Can you work these out from the model? Positions are in its coordinate system, mm. Face numbers are marked on the shaded views. Round coordinates to 2 decimals unless told otherwise and drop trailing zeros. Loops run counter-clockwise (first coordinate to the right, second up) from the corner with the lowest first, then second, coordinate; pieces in that order, holes last. Notation, with made-up numbers: (-31, 2) -> (-4, 2) arc R16 cw to (-4, 26) -> close; hole circle Ø6 at (88.25, -16). An arc over 180 degrees is marked (long way). Answer as a JSON object with one key per item and string values.
```python
from build123d import *

# Parameters (mm, degrees)
PAD009_DEPTH          = 2
SKETCH015_R           = 2
POCKET005_DEPTH       = 2
POCKET006_DEPTH       = 2
PAD010_DEPTH          = 160
POLARPATTERN001_COUNT = 6
SKETCH018_W           = 8
SKETCH018_H           = 3
POCKET007_DEPTH       = 2
POLARPATTERN002_COUNT = 6
SKETCH019_W           = 14
SKETCH019_H           = 27
PAD011_DEPTH          = 3
POLARPATTERN003_COUNT = 6
POCKET008_DEPTH       = 5
POLARPATTERN004_COUNT = 6
SKETCH021_R           = 50
SKETCH021_R_2         = 46
PAD012_DEPTH          = 6
SKETCH022_W           = 4
SKETCH022_H           = 3
POCKET009_DEPTH       = 6
POLARPATTERN005_COUNT = 4
SKETCH023_W           = 2.5
SKETCH023_H           = 3
POLARPATTERN006_COUNT = 4
POCKET010_DEPTH       = 5


with BuildPart() as part:
    # Sketch014 → Pad009 (new body)
    with BuildSketch(Plane.XY):
        with BuildLine():
            Line((-52, -60), (52, -60))
            ThreePointArc((52, -60), (57.6568542495, -57.6568542495), (60, -52))
            Line((60, -52), (60, 52))
            ThreePointArc((60, 52), (57.6568542495, 57.6568542495), (52, 60))
            Line((52, 60), (-52, 60))
            ThreePointArc((-52, 60), (-57.6568542495, 57.6568542495), (-60, 52))
            Line((-60, 52), (-60, -52))
            ThreePointArc((-60, -52), (-57.6568542495, -57.6568542495), (-52, -60))
        make_face()
    extrude(amount=PAD009_DEPTH)

    # Sketch015 (on Face10 of Pad009) → Pocket005 (cut)
    with BuildSketch(Plane.XY.offset(2)):
        with Locations((-52, 52)):
            Circle(SKETCH015_R)
        with Locations((52, 52)):
            Circle(SKETCH015_R)
        with Locations((52, -52)):
            Circle(SKETCH015_R)
        with Locations((-52, -52)):
            Circle(SKETCH015_R)
    extrude(amount=-POCKET005_DEPTH, mode=Mode.SUBTRACT)

    # Sketch016 (on Face5 of Pocket005) → Pocket006 (cut)
    with BuildSketch(Plane.XY.offset(2)):
        Polygon((30, 0), (15, 25.9807621135), (-15, 25.9807621135), (-30, 0), (-15, -25.9807621135), (15, -25.9807621135), align=None)
    extrude(amount=-POCKET006_DEPTH, mode=Mode.SUBTRACT)

    # Sketch017 (on Face5 of Pocket006) → Pad010 (join)
    with BuildSketch(Plane.XY.offset(2)):
        Polygon((-7, 26), (7, 26), (7, 29), (5, 29), (5, 27.5), (-5, 27.5), (-5, 29), (-7, 29), align=None)
    pad010 = extrude(amount=PAD010_DEPTH)

    # PolarPattern001: Pad010 ×6 about axis
    polarpattern001_axis = Axis((0, 0, 2), (0, 0, 1))
    for i in range(1, POLARPATTERN001_COUNT):
        add(pad010.rotate(polarpattern001_axis, i * 360 / POLARPATTERN001_COUNT))

    # Sketch018 (on Face5 of PolarPattern001) → Pocket007 (cut)
    with BuildSketch(Plane.XY.offset(2)):
        with Locations((0, 30)):
            Rectangle(SKETCH018_W, SKETCH018_H)
    pocket007 = extrude(amount=-POCKET007_DEPTH, mode=Mode.SUBTRACT)

    # PolarPattern002: Pocket007 ×6 about axis
    polarpattern002_axis = Axis((0, 0, 2), (0, 0, 1))
    for i in range(1, POLARPATTERN002_COUNT):
        add(pocket007.rotate(polarpattern002_axis, i * 360 / POLARPATTERN002_COUNT), mode=Mode.SUBTRACT)

    # Sketch019 (on Face98 of PolarPattern002) → Pad011 (join)
    with BuildSketch(Plane.XY.offset(162)):
        with Locations((0, 13.5)):
            Rectangle(SKETCH019_W, SKETCH019_H)
    pad011 = extrude(amount=-PAD011_DEPTH)

    # PolarPattern003: Pad011 ×6 about axis
    polarpattern003_axis = Axis((0, 0, 162), (0, 0, 1))
    for i in range(1, POLARPATTERN003_COUNT):
        add(pad011.rotate(polarpattern003_axis, i * 360 / POLARPATTERN003_COUNT))

    # Sketch020 (on Face71 of PolarPattern003) → Pocket008 (cut)
    with BuildSketch(Plane(origin=(23.8156986041, 13.75, 0), x_dir=(-0.5, 0.8660254038, 0), z_dir=(0.8660254038, 0.5, 0))):
        Polygon((2.9997494237, 155.3827539752), (1.5334536671, 158), (-1.4662957566, 158.0387736377), (-2.9997494237, 155.4603012506), (-1.5334536671, 152.8430552259), (1.4662957566, 152.8042815882), align=None)
    pocket008 = extrude(amount=-POCKET008_DEPTH, mode=Mode.SUBTRACT)

    # PolarPattern004: Pocket008 ×6 about axis
    polarpattern004_axis = Axis((0, 0, 0), (0, 0, 1))
    for i in range(1, POLARPATTERN004_COUNT):
        add(pocket008.rotate(polarpattern004_axis, i * 360 / POLARPATTERN004_COUNT), mode=Mode.SUBTRACT)

    # Sketch021 (on Face5 of PolarPattern004) → Pad012 (join)
    with BuildSketch(Plane.XY.offset(2)):
        Circle(SKETCH021_R)
        Circle(SKETCH021_R_2, mode=Mode.SUBTRACT)
    extrude(amount=PAD012_DEPTH)

    # Sketch022 (on Face47 of Pad012) → Pocket009 (cut)
    with BuildSketch(Plane.XY.offset(8)):
        with Locations((0, -49)):
            Rectangle(SKETCH022_W, SKETCH022_H)
    pocket009 = extrude(amount=-POCKET009_DEPTH, mode=Mode.SUBTRACT)

    # PolarPattern005: Pocket009 ×4 about axis
    polarpattern005_axis = Axis((0, 0, 8), (0, 0, 1))
    for i in range(1, POLARPATTERN005_COUNT):
        add(pocket009.rotate(polarpattern005_axis, i * 360 / POLARPATTERN005_COUNT), mode=Mode.SUBTRACT)

    # SubtractivePipe: sweep along a path in Sketch024
    with BuildLine(Plane.XY.offset(2)) as subtractivepipe_path:
        ThreePointArc((-12.940932525, -48.2962966011), (-6.5262994853, -49.5722444018), (0, -50))
    # Sketch023 (on DatumPlane) → SubtractivePipe (sweep, cut)
    with BuildSketch(Plane.YZ.offset(-2)):
        with Locations((-48.7099839872, 3.5)):
            Rectangle(SKETCH023_W, SKETCH023_H)
    subtractivepipe = sweep(path=subtractivepipe_path.line, mode=Mode.SUBTRACT)

    # PolarPattern006: SubtractivePipe ×4 about axis
    polarpattern006_axis = Axis((0, 0, 0), (0, 0, 1))
    for i in range(1, POLARPATTERN006_COUNT):
        add(subtractivepipe.rotate(polarpattern006_axis, i * 360 / POLARPATTERN006_COUNT), mode=Mode.SUBTRACT)

    # Sketch025 (on Face123 of PolarPattern006) → Pocket010 (cut)
    with BuildSketch(Plane.XY.offset(162)):
        Polygon((6.9282031151, 4.0000001994), (-2.303e-07, 8), (-6.9282033454, 3.9999998006), (-6.9282031151, -4.0000001994), (2.303e-07, -8), (6.9282033454, -3.9999998006), align=None)
    extrude(amount=-POCKET010_DEPTH, mode=Mode.SUBTRACT)


with BuildPart() as part_1:
    # Body002 placement: moved
    add(part.part.moved(Location((0, 0, 61.6))))


solid = part_1.part
```
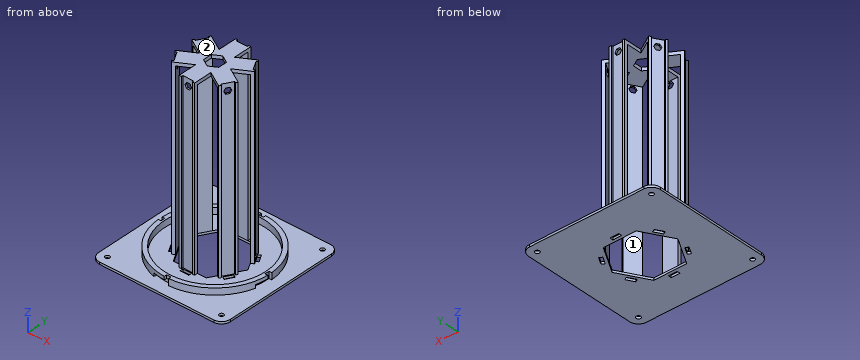
Q1. If I drill on L1, parallel to Y at x = -52, z = 62.3; L2, parallel to Y at x = 0, z = 65.7; L3, parallel to Z at x = 17, y = 33, over which ranges is the centre line in solid material (lowest first)? Write a range as [from, to].
Determined:
{"L1": "[-60, -54], [-50, 50], [54, 60]", "L2": "[-47.5, -46], [-27.5, -26], [26, 27.5], [46, 47.5]", "L3": "[61.6, 63.6]"}
Q2. I want a section at C-C, the plane x = -43.5. Write out the boundary of the cut face in (y, z).
Determined:
{"outline": "(-60, 61.6) -> (60, 61.6) -> (60, 63.6) -> (24.65, 63.6) -> (24.65, 69.6) -> (14.96, 69.6) -> (14.96, 63.6) -> (-14.96, 63.6) -> (-14.96, 69.6) -> (-24.65, 69.6) -> (-24.65, 63.6) -> (-60, 63.6) -> close"}
Q3. We'd pull the mould along Y, two halves only. Please class the marked faces 1 and 2: pulls with the +Y half, pulls with the -Y half, needs draft (parallel to the pull), parting line crosses it, or undercut.
Determined:
{"face 1": "undercut", "face 2": "needs draft"}
Q4. I want a section at B-B, the plane y = 38.5. Write out the boundary of the cut face in (x, z), then the cut area to 3 significant figures.
Determined:
{"outline": "(-60, 61.6) -> (60, 61.6) -> (60, 63.6) -> (31.9, 63.6) -> (31.9, 69.6) -> (25.17, 69.6) -> (25.17, 63.6) -> (-25.17, 63.6) -> (-25.17, 69.6) -> (-31.9, 69.6) -> (-31.9, 63.6) -> (-60, 63.6) -> close", "area": "321 mm²"}
Q5. I want a section at A-A, the plane z = 200. Give the number of separate pieces and of enclosed holes in the cut face, then the cut area to 3 significant figures.
Determined:
{"separate pieces": "6", "enclosed holes": "0", "area": "162 mm²"}
Q6. I'm going to push flat-ended pins straight in: pin 1 (4.5 mm diameter, centred on x = -52, y = -52, fed in from +Z); pin 2 (1 mm diameter, centred on x = -24.5, z = 204, fed in from +Y); pin 3 (8 mm diameter, centred on y = 24, z = 166, fed in from -X); pin 4 (6 mm diameter, centred on x = 11.5, z = 154, fed in from +Y). Where does each tip first touch, or does it pass through?
Determined:
{"pin 1": "z = 63.6", "pin 2": "y = 13.43", "pin 3": "x = -21.94", "pin 4": "through"}
